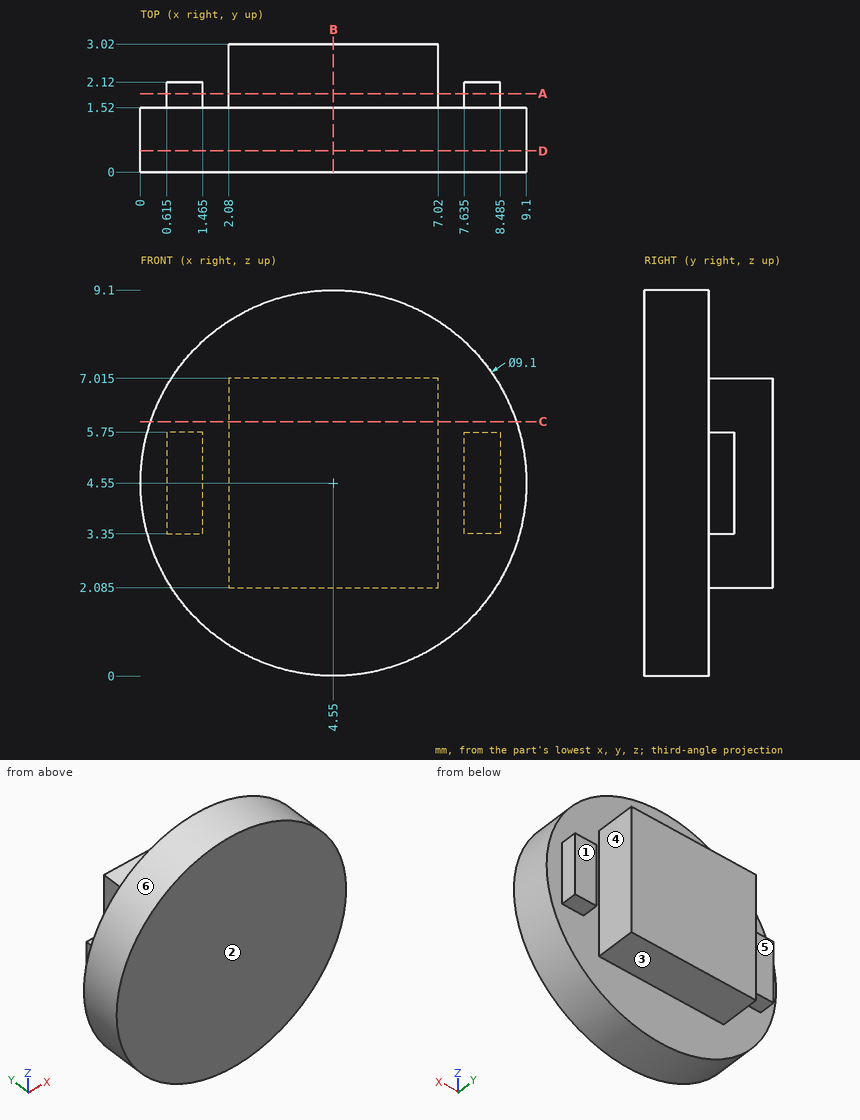
Here's the drawing with two shaded views (mm, measured from the low corner). I have some questions. A direction names the side the tool comes from. Give positions to 0.01 mm unless a question says otherwise; leave off trailing zeros. Order: outer loops, then holes, each group sorted by start corner. A loop starts at its lowest first (then second) coordinate and runs counter-clockwise, first axis right, second up. Notation, with made-up numbers: M 9.5,-11 L 62.5,-11 A37 ccw 62.5,26 Z; hole C -10,63 d5. An arc over 180 degrees is marked long. Answer as a JSON object with one key per item and string values. Group by question number.
1) Please list where these lines run through material, in increasing order: L1, parallel to X at y = 2.05, z = 4 (3 decimals); L2, parallel to Z at x = 6.75, y = 2.15 (3 decimals); L3, parallel to X at y = 2.6, z = 5.25. Write a range as [from, to].
2) We'd pull the mould along X, two halves only. Please class the marked faces 4, 5 and 6: pulls with the +X half, pulls with the -X half, needs draft (parallel to the pull), parting line crosses it, or undercut.
3) I'm going to push flat-ended pins straight in: pin 1 Ø0.9 at (x, z) = (1, 4) entering from +Y; pin 2 Ø0.5 at (y, z) = (1.5, 4) entering from +X; pin 3 Ø0.8 at (y, z) = (2, 5.5) entering from -X (3 decimals). Where does each tip first touch, or does it pass through?
4) Suppose I cut it at B-B, the plane x = 4.55. Write out the boundary of the cut face in (y, z) (3 decimals).
5) Suppose I cut it at D-D, the plane y = 0.5. Write out the boundary of the cut face in (x, z), plus the area to 3 significant figures.
6) Suppose I cut it at C-C, the plane z = 6. Write out the boundary of the cut face in (x, y), plus the area to 3 significant figures.
7) Suppose I cut it at A-A, the plane y = 1.85. Write out the boundary of the cut face in (x, z) (3 decimals).
8) On a 3-axis mill with a long thin cutter (end or side, diameter ignored), from which of +Z, -Z, +X, -X, +Y, -Y can I reach the whole of each face in a straight line? I mean the marked faces 1, 2 and 3. Say none if no direction works.
Results found:
{
 "1": {"L1": "[0.615, 1.465], [2.08, 7.02], [7.635, 8.485]", "L2": "[2.085, 7.015]", "L3": "[2.08, 7.02]"},
 "2": {"face 4": "undercut", "face 5": "needs draft", "face 6": "parting line crosses it"},
 "3": {"pin 1": "y = 2.12", "pin 2": "x = 9.09", "pin 3": "x = 0.615"},
 "4": {"outline": "M 0,0 L 1.52,0 L 1.52,2.085 L 3.02,2.085 L 3.02,7.015 L 1.52,7.015 L 1.52,9.1 L 0,9.1 Z"},
 "5": {"outline": "C 4.55,4.55 d9.1", "area": "65.0 mm²"},
 "6": {"outline": "M 0.24,0 L 8.86,0 L 8.86,1.52 L 7.02,1.52 L 7.02,3.02 L 2.08,3.02 L 2.08,1.52 L 0.24,1.52 Z", "area": "20.5 mm²"},
 "7": {"outline": "M 0.615,3.35 L 1.465,3.35 L 1.465,5.75 L 0.615,5.75 Z; M 2.08,2.085 L 7.02,2.085 L 7.02,7.015 L 2.08,7.015 Z; M 7.635,3.35 L 8.485,3.35 L 8.485,5.75 L 7.635,5.75 Z"},
 "8": {"face 1": "+Z, -Z, +X, +Y", "face 2": "+Z, -Z, +X, -X, -Y", "face 3": "-Z, +X, -X, +Y"}
}
